The listing builds one solid part. Answer for the finished solid, in the listing's coordinates (mm). A direction names the side the tool comes from. Give positions to 0.01 mm unless a question says otherwise; leave off trailing zeros. Loops run counter-clockwise (first coordinate to the right, second up) from the corner with the lowest first, then second, coordinate; pieces in that order, holes last.
Item 1: The mould has two halves that part along Z. Classify faces 5 (the face through (-5, 1, 16)), 6 (the face through (-19.95, 2, 0)), 7 (the face through (-39.1, 1.27, -15.14)), 8 (the face through (2.683, 2, 14)): pulls with the +Z half, pulls with the -Z half, needs draft (parallel to the pull), parting line crosses it, or undercut.
Item 2: Section A-A, the plane x = 26 is taken. Give the vertices of the cut face in (y, z), and give its area (3 significant figures).
Item 3: Section D-D, the plane y = 0.5 is taken. Give the number of separate pieces and of enclosed holes in the cut face, and give its area (3 significant figures).
Item 4: Section C-C, the plane x = 7 is taken. Give the vertices of the cut face in (y, z).
Item 5: A tool of negligible diameter and unlimited length cuts with its end or side. For faces 1 (the face through (-18, 2, -7.811)), 2 (the face through (4.66, 1.23, -10)), 3 (the face through (12, 2, -11.25)), 4 (the face through (21.716, 2, 14)), from which of +Z, -Z, +X, -X, +Y, -Y can it reach the whole face along a straight path? Write none if from no direction.
Item 6: Section B-B, the plane z = -3.5 is taken. Give the vertices of the cut face in (x, y).
Item 7: Each of these flat-tipped pins is pushed along its axis until it touches: pin 1 Ø1.2 at (y, z) = (1.5, 14.5) entering from -X; pin 2 Ø1.4 at (x, z) = (-3, -1.5) entering from +Y; pin 3 Ø0.8 at (y, z) = (1.5, 14) entering from +X. Where does it stop, or does it pass through?
Item 8: Consider line 1 along X through (y, z) = (1.6, -7); line 2 along X through (y, z) = (1.2, 8.75); line 3 along X through (y, z) = (1.7, -13.25). Determine where each line is inside the solid, lowest interval first.
from build123d import *

# Parameters (mm, degrees)
SKETCH1_R           = 1.6
SKETCH1_R_2         = 1.25
BOSS_EXTRUDE1_DEPTH = 2.5
SKETCH4_W           = 4.046420923
SKETCH4_H           = 15.954838713
SKETCH4_W_2         = 4.570038916
SKETCH4_H_2         = 16.10433934
SKETCH4_W_3         = 19.288754193
SKETCH4_H_3         = 4.75
SKETCH4_W_4         = 19.033274005
CUT_EXTRUDE2_DEPTH  = 1.5
FILLET1_R           = 3


with BuildPart() as part:
    # Sketch1 → Boss-Extrude1 (new body)
    with BuildSketch(Plane(origin=(0, 0, 0), x_dir=(1, 0, 0), z_dir=(0, 1, 0))):
        Polygon((-30, -16), (30, -16), (30, 16), (-30, 16), (-40, 16), (-40, -16), align=None)
        with Locations(Location((-26, 12, 0), (0, 0, 270))):
            Circle(SKETCH1_R, mode=Mode.SUBTRACT)
        with Locations(Location((26, 12, 0), (0, 0, 270))):
            Circle(SKETCH1_R, mode=Mode.SUBTRACT)
        with Locations(Location((26, -12, 0), (0, 0, 270))):
            Circle(SKETCH1_R, mode=Mode.SUBTRACT)
        with Locations(Location((-26, -12, 0), (0, 0, 270))):
            Circle(SKETCH1_R, mode=Mode.SUBTRACT)
        with Locations(Location((-18.554722835, 9.82, 0), (0, 0, 270))):
            Circle(SKETCH1_R_2, mode=Mode.SUBTRACT)
        with Locations(Location((-3.314722835, 9.82, 0), (0, 0, 270))):
            Circle(SKETCH1_R_2, mode=Mode.SUBTRACT)
        with Locations(Location((-3.314722835, -10.5, 0), (0, 0, 270))):
            Circle(SKETCH1_R_2, mode=Mode.SUBTRACT)
        with Locations(Location((-18.554722835, -10.5, 0), (0, 0, 270))):
            Circle(SKETCH1_R_2, mode=Mode.SUBTRACT)
        with Locations(Location((4.60621428, 8.75, 0), (0, 0, 270))):
            Circle(SKETCH1_R_2, mode=Mode.SUBTRACT)
        with Locations(Location((19.20621428, 8.75, 0), (0, 0, 270))):
            Circle(SKETCH1_R_2, mode=Mode.SUBTRACT)
        with Locations(Location((19.20621428, -8.75, 0), (0, 0, 270))):
            Circle(SKETCH1_R_2, mode=Mode.SUBTRACT)
        with Locations(Location((4.60621428, -8.75, 0), (0, 0, 270))):
            Circle(SKETCH1_R_2, mode=Mode.SUBTRACT)
        with Locations(Location((-34, 13.25, 0), (0, 0, 270))):
            Circle(SKETCH1_R_2, mode=Mode.SUBTRACT)
        with Locations(Location((-34, -13.25, 0), (0, 0, 270))):
            Circle(SKETCH1_R_2, mode=Mode.SUBTRACT)
    extrude(amount=BOSS_EXTRUDE1_DEPTH)

    # Sketch4 → Cut-Extrude2 (cut)
    with BuildSketch(Plane(origin=(0, 2.5, 0), x_dir=(1, 0, 0), z_dir=(0, 1, 0))):
        with Locations((-17.926852164, -0.166011636)):
            Rectangle(SKETCH4_W, SKETCH4_H)
        with Locations((-3.846505054, -0.091261322)):
            Rectangle(SKETCH4_W_2, SKETCH4_H_2)
        with Locations((11.879828742, 13.625)):
            Rectangle(SKETCH4_W_3, SKETCH4_H_3)
        with Locations((12.199178977, -13.625)):
            Rectangle(SKETCH4_W_4, SKETCH4_H_3)
    extrude(amount=-CUT_EXTRUDE2_DEPTH, mode=Mode.SUBTRACT)

    # Fillet1
    fillet1_edges = [part.edges().sort_by_distance(p)[0] for p in [
        (30, 1.25, 16),
        (-40, 1.25, 16),
        (-40, 1.25, -16),
        (30, 1.25, -16),
    ]]
    fillet(fillet1_edges, radius=FILLET1_R)


solid = part.part
Worked answers:
1. face 5: pulls with the +Z half
1. face 6: undercut
1. face 7: pulls with the -Z half
1. face 8: needs draft
2. outline: (0, -16) - (2.5, -16) - (2.5, -13.6) - (0, -13.6) - close; (0, -10.4) - (2.5, -10.4) - (2.5, 10.4) - (0, 10.4) - close; (0, 13.6) - (2.5, 13.6) - (2.5, 16) - (0, 16) - close
2. area: 64.0 mm2
3. separate pieces: 1
3. enclosed holes: 14
3. area: 2,150 mm2
4. outline: (0, -16) - (1, -16) - (1, -11.25) - (2.5, -11.25) - (2.5, 11.25) - (1, 11.25) - (1, 16) - (0, 16) - close
5. face 1: +Y
5. face 2: +Y, -Y
5. face 3: -Z, +Y
5. face 4: +Z, +Y
6. outline: (-40, 0) - (30, 0) - (30, 2.5) - (-1.56, 2.5) - (-1.56, 1) - (-6.13, 1) - (-6.13, 2.5) - (-15.9, 2.5) - (-15.9, 1) - (-19.95, 1) - (-19.95, 2.5) - (-40, 2.5) - close
7. pin 1: stops at x = -39.86
7. pin 2: stops at y = 1
7. pin 3: stops at x = 29.94
8. line 1: x = -40 to -19.95, -15.9 to -6.13, -1.56 to 30
8. line 2: x = -40 to 3.36, 5.86 to 17.96, 20.46 to 30
8. line 3: x = -39.99 to -35.25, -32.75 to -27, -25 to 2.24, 21.52 to 25, 27 to 29.99
